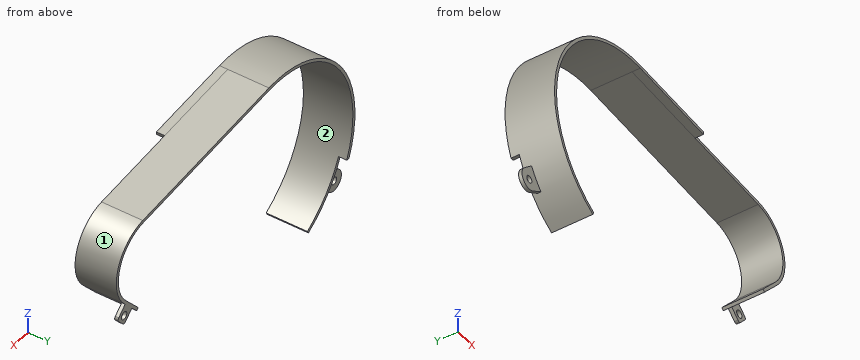
from build123d import *
from build123d.topology import SkipClean

# Parameters (mm, degrees)
BASE_FLANGE1_DEPTH  = 38.1
CUT_EXTRUDE1_DEPTH  = 7.62
BOSS_EXTRUDE1_DEPTH = 3.175
BOSS_EXTRUDE2_DEPTH = 7.62
SKETCH11_R          = 3.5
BOSS_EXTRUDE3_DEPTH = 3.175


# Sheet-metal steps are written as plain solids
with BuildPart() as part:
    # Sketch1 → Base-Flange1 (new body)
    with BuildSketch(Plane(origin=(0, 0, 0), x_dir=(1, 0, 0), z_dir=(0, 1, 0))):
        with BuildLine():
            Line((-658.18839, -181.815019342), (-493.414651072, -163.065661223))
            ThreePointArc((-493.414651072, -163.065661223), (-463.516823985, -139.706651468), (-470.767754496, -102.464908652))
            Line((-470.767754496, -102.464908652), (-487.062469778, -84.698684743))
            Line((-487.062469778, -84.698684743), (-485.096976273, -82.895985576))
            Line((-485.096976273, -82.895985576), (-468.802260992, -100.662209486))
            ThreePointArc((-468.802260992, -100.662209486), (-461.018573288, -140.640264051), (-493.113122906, -165.715561177))
            Line((-493.113122906, -165.715561177), (-657.886861835, -184.464919296))
            ThreePointArc((-657.886861835, -184.464919296), (-764.999542035, -116.070482162), (-720.157705771, 2.841817501))
            Line((-720.157705771, 2.841817501), (-718.812633408, 0.538847823))
            ThreePointArc((-718.812633408, 0.538847823), (-762.468736724, -115.229106217), (-658.18839, -181.815019342))
        make_face()
    extrude(amount=-BASE_FLANGE1_DEPTH)

    # Sketch7 → Cut-Extrude1 (cut)
    with BuildSketch(Plane(origin=(-720.157705771, 0, -2.841817501), x_dir=(1, 0, 0), z_dir=(0, 1, 0))):
        with BuildLine():
            Line((1.345072363, -2.302969678), (0, 0))
            ThreePointArc((0, 0), (-25.04555192, -20.685894616), (-42.216883241, -48.26))
            Line((-42.216883241, -48.26), (-39.320240627, -48.26))
            ThreePointArc((-39.320240627, -48.26), (-22.669860727, -22.023203588), (1.345072363, -2.302969678))
        make_face()
    extrude(amount=-CUT_EXTRUDE1_DEPTH, mode=Mode.SUBTRACT)

    # Sketch9 → Boss-Extrude1 (add)
    with BuildSketch(Plane(origin=(0, -11.93175668, 0), x_dir=(1, 0, 0), z_dir=(0, 1, 0))):
        with BuildLine():
            Line((-766.021160844, -26.574153948), (-756.947378036, -34.362103973))
            ThreePointArc((-756.947378036, -34.362103973), (-751.259248381, -25.482371354), (-744.675064761, -17.245078325))
            Line((-744.675064761, -17.245078325), (-754.96335975, -11.151090609))
            ThreePointArc((-754.96335975, -11.151090609), (-767.558577165, -13.796318349), (-766.021160844, -26.574153948))
        make_face()
        with BuildLine():
            ThreePointArc((-761.982172567, -21.837237166), (-757.32668993, -21.510922268), (-757.653004828, -16.85543963))
            ThreePointArc((-757.653004828, -16.85543963), (-762.308487465, -17.181754528), (-761.982172567, -21.837237166))
        make_face(mode=Mode.SUBTRACT)
    extrude(amount=-BOSS_EXTRUDE1_DEPTH)

    # Sketch10 → Boss-Extrude2 (add)
    with SkipClean():  # the faces are left unmerged after this step: merging them gives an invalid solid
        with BuildSketch(Plane.XZ.offset(38.1)):
            with BuildLine():
                Line((-718.812633408, -0.538847823), (-720.157705771, -2.841817501))
                ThreePointArc((-720.157705771, -2.841817501), (-764.999542035, 116.070482162), (-657.886861835, 184.464919296))
                Line((-657.886861835, 184.464919296), (-575.49999237, 175.090240236))
                Line((-575.49999237, 175.090240236), (-575.801520536, 172.440340282))
                Line((-575.801520536, 172.440340282), (-658.18839, 181.815019342))
                ThreePointArc((-658.18839, 181.815019342), (-762.468736724, 115.229106217), (-718.812633408, -0.538847823))
            make_face()
        extrude(amount=BOSS_EXTRUDE2_DEPTH)

    # Sketch11 → Boss-Extrude3 (add)
    with SkipClean():  # the faces are left unmerged after this step: merging them gives an invalid solid
        with BuildSketch(Plane(origin=(0, 0, 0), x_dir=(1, 0, 0), z_dir=(0, 1, 0))):
            with BuildLine():
                Line((-470.547014649, -82.037691541), (-478.876963309, -89.677702295))
                Line((-478.876963309, -89.677702295), (-470.089903254, -99.258285554))
                Line((-470.089903254, -99.258285554), (-461.759954594, -91.618274801))
                ThreePointArc((-461.759954594, -91.618274801), (-460.939178, -89.856007635), (-461.604912368, -88.029519876))
                Line((-461.604912368, -88.029519876), (-466.958259724, -82.192733767))
                ThreePointArc((-466.958259724, -82.192733767), (-468.72052689, -81.371957173), (-470.547014649, -82.037691541))
            make_face()
            with Locations(Location((-468.787614295, -89.074866795, 0), (0, 0, 270))):
                Circle(SKETCH11_R, mode=Mode.SUBTRACT)
        extrude(amount=-BOSS_EXTRUDE3_DEPTH)


solid = part.part
Design review of the part built by this model. Coordinates are the model's own, in mm. Face numbers are marked on the shaded views. Round coordinates to 2 decimals unless told otherwise and drop trailing zeros. Loops run counter-clockwise (first coordinate to the right, second up) from the corner with the lowest first, then second, coordinate; pieces in that order, holes last. Notation, with made-up numbers: (-38, 57.25) - (-28, 57.25) arc R25 ccw to (-28, 72.25) - close; hole circle Ø4 at (11, 57.5). An arc over 180 degrees is marked (long way). One line per question, with ' | ' between items.
1. We need section B-B, the plane x = -734. State the section outline as (y, z) points, and give its area (3 significant figures).
Results are:
outline: (-45.72, 6.89) - (-7.62, 6.89) - (-7.62, 10.4) - (-45.72, 10.4) - close; (-45.72, 158.11) - (0, 158.11) - (0, 161.62) - (-45.72, 161.62) - close | area: 294 mm²
2. Draft analysis for pull direction X (two halves, no side actions). For the marked faces 1 and 2, state which applies: released by +X, released by -X, zero draft, split by the parting line, or undercut.
Results are:
face 1: released by +X | face 2: undercut
3. We need section D-D, the plane x = -645.5. State the section outline as (y, z) points.
Results are:
outline: (-45.72, 180.37) - (0, 180.37) - (0, 183.06) - (-45.72, 183.06) - close
4. We need section A-A, the plane z = 155. State the section outline as (x, y) points, and give its area (3 significant figures).
Results are:
outline: (-741.17, -45.72) - (-737.38, -45.72) - (-737.38, 0) - (-741.17, 0) - close; (-474.42, -38.1) - (-470.42, -38.1) - (-470.42, 0) - (-474.42, 0) - close | area: 326 mm²
5. For L1, parallel to Z at x = -671, y = -41; L2, parallel to Z at x = -666, y = -40; L3, parallel to X at y = -43, z = 87, list the stretches that pass through material, from the lowest coordinate up. Write a range as [from, to].
Results are:
L1: z = [182.43, 185.1] | L2: z = [182.39, 185.06] | L3: x = [-770.11, -767.44]
6. Clearance check with flat-ended pins moving along their axes: P1, Ø1.5, axis at x = -717.5, y = -8, coming from the -Z side; P2, Ø2.5, axis at x = -761.5, y = -4, coming from the -Z side; P3, Ø5, axis at x = -729, y = -28.5, coming from the +Z side; P4, Ø6.5, axis at x = -468.79, z = 89.07, coming from the +Y side. State where each tip first meets the part, or that it passes through.
Results are:
P1: stops at z = 169.37 | P2: stops at z = 45.42 | P3: stops at z = 167.32 | P4: passes through
7. We need section C-C, the plane y = -30. State the section outline as (x, z) points, and give its area (3 significant figures).
Results are:
outline: (-720.16, -2.84) - (-718.81, -0.54) arc R98.19 cw to (-658.19, 181.82) - (-493.41, 163.07) arc R36.3 cw to (-470.77, 102.46) - (-487.06, 84.7) - (-485.1, 82.9) - (-468.8, 100.66) arc R38.97 ccw to (-493.11, 165.72) - (-657.89, 184.46) arc R100.86 ccw to start | area: 1,450 mm²
